Part print with two shaded views. Sizes in mm from the minimum x, y, z corner. Round coordinates to 2 decimals unless told otherwise and drop trailing zeros. Loops run counter-clockwise (first coordinate to the right, second up) from the corner with the lowest first, then second, coordinate; pieces in that order, holes last. Notation, with made-up numbers: (21, 47) - (43, 47) arc R26 cw to (43, 77) - close; hole circle Ø1 at (43, 45.5). An arc over 180 degrees is marked (long way). Write each question's results on one line, items separated by ' | '. Start each with the question number.
(1) Drill centre lines: L1, parallel to Y at x = 25, z = 4.5 (1 decimal); L2, parallel to X at y = 3.75, z = 14.75; L3, parallel to X at y = 5, z = 3 (1 decimal). Where is each one in solid material? Low to high.
(2) Cut at C-C, the plane z = 18. List the corners of the cut face in (x, y), then the cut area to 3 significant figures.
(3) Flat gauge pins, fed straight in: P1, Ø4, axis at y = 8.5, z = 14, coming from the -X side; P2, Ø1.5, axis at y = 1.5, z = 4, coming from the -X side; P3, Ø1, axis at y = 7.5, z = 11, coming from the +X side. Where does each tip first touch, or does it go through?
(4) Mould opens along X. For the marked faces 1, 2 and 3 say: released by +X, released by -X, zero draft, split by the parting line, or undercut.
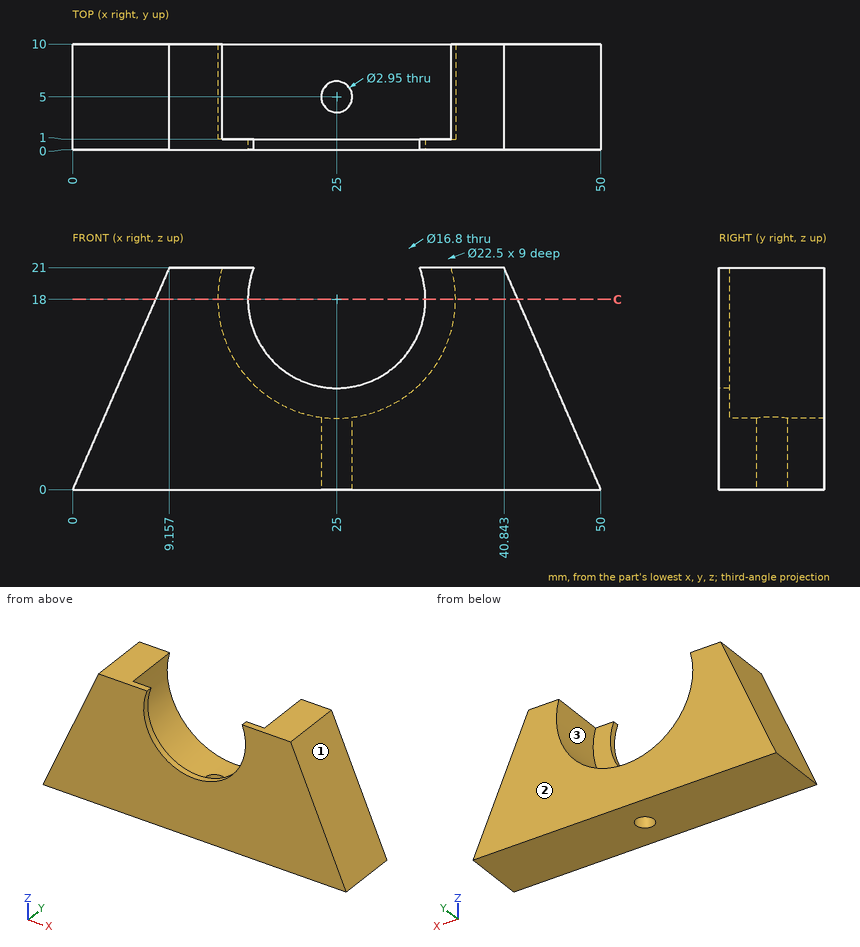
A:
1) L1: 0 to 3.5, 6.5 to 10 | L2: 6.43 to 14.23, 35.77 to 43.57 | L3: 1.3 to 23.5, 26.5 to 48.7
2) outline: (7.85, 0) - (16.6, 0) - (16.6, 1) - (13.75, 1) - (13.75, 10) - (7.85, 10) - close; (33.4, 0) - (42.15, 0) - (42.15, 10) - (36.25, 10) - (36.25, 1) - (33.4, 1) - close | area: 124 mm2
3) P1: x = 5.23 | P2: x = 1.42 | P3: x = 45.42
4) face 1: released by +X | face 2: zero draft | face 3: undercut
